Build history of the part. All positions in model axes, mm. Face numbers are marked on the shaded views. A direction names the side the tool comes from. Give positions to 0.01 mm unless a question says otherwise; leave off trailing zeros. Write each loop counter-clockwise with the first axis right and the second up, starting at its lowest first coordinate (ties: lowest second). Pieces come first, ordered by that corner, then holes. Notation, with made-up numbers: (-27, 1) -> (-11, 1) arc R36 ccw to (-11, 35) -> close; hole circle Ø7 at (34.25, -26.5). An arc over 180 degrees is marked (long way). Write item = value, one per line. Start each with the question number.
Q1. Saw through at A-A, the plane z = 0. List the corners of the cut face in (x, y).
Q2. Drop flat-ended pins along their axis: P1, Ø2, axis at x = 6.5, z = 0.5, coming from the -Y side; P2, Ø3, axis at x = 3, z = 0, coming from the +Y side; P3, Ø3, axis at y = 0, z = -1.5, coming from the +X side; P4, Ø2, axis at x = 6, y = 0, coming from the +Z side. Give the stop position or say it passes through.
Q3. Saw through at C-C, the plane x = 7. List the corners of the cut face in (y, z).
Q4. Mould opens along X. For the marked faces 1, 2, 3 and 4 say: pulls with the +X half, pulls with the -X half, needs draft (parallel to the pull), parting line crosses it, or undercut.
Q5. Saw through at B-B, the plane y = 0. List the corners of the cut face in (x, z), then the cut area to 3 significant figures.
Q6. Wall check: line 1 (X direction, y = 0.25, z = 1.05); line 2 (X direction, y = 0.05, z = 2.05); line 3 (Z direction, x = 3.25, y = 0.1). Give the ranges that are in metal, low to high.
Q7. Tool access for the marked faces 5 and 6: list every direction of +Z, -Z, +X, -X, +Y, -Y with a clear straight run to the whole face (end or side of a thin tool).
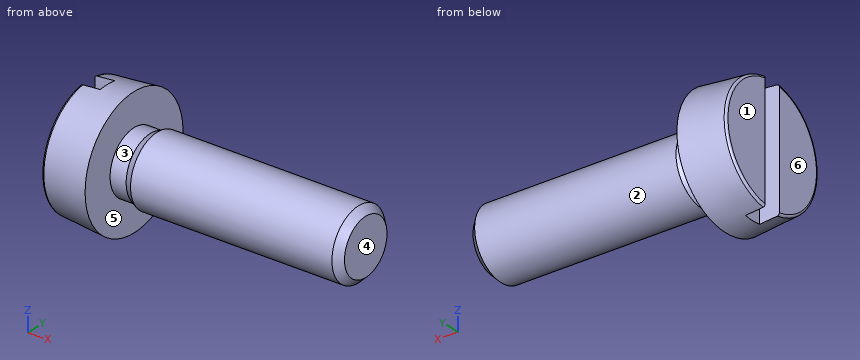
Autodesk Inventor part; units mm, degrees
ref_plane "Work Plane1" through (30.1625, 0, 0) normal (0, 0, -1) x (1, 0, 0)
ref_plane "YZ Plane" through (0, 0, 0) normal (1, 0, 0) x (0, 1, 0)
ref_plane "XZ Plane" through (0, 0, 0) normal (0, 1, 0) x (-1, 0, 0)
sketch "Szkic1" plane through (0, 0, 0) normal (0, 0, 1) x (1, 0, 0)
  line L0 (-2, 0) -> (10, 0)
  line L1 (10, 0) -> (10, 1.5)
  line L2 (10, 1.5) -> (1, 1.5)
  line L3 (1, 1.5) -> (0.6932, 1.3467)
  line L4 (0.6932, 1.3467) -> (0, 1.3467)
  line L5 (0, 1.3467) -> (0, 2.75)
  line L6 (-4.4, 0) -> (12.4, 0)
  line L7 (0, -0.55) -> (0, 3.3)
  line L8 (-2, 0) -> (-2, 2.575)
  line L9 (0, 2.75) -> (-2, 2.575)
  line L10 (1, 1.5) -> (0, 1.5) construction
  dimension "d0" = 10
  dimension "d1" = 9
  dimension "d2" = 0.3068
  dimension "d3" = 2
  dimension "d4" = 3
  dimension "d5" = 2.6935
  dimension "d9" = 5.5
  dimension "d10" = 5
revolve "Bryła" add sketch "Szkic1" angle 360 about axis through (-2, 0, 0) along (1, 0, 0)
sketch "Szkic2" plane through (-2, 0, 0) normal (-1, 0, 0) x (0, 0, 1)
  circle A0 centre (0, 0) radius 2.75
  line L0 (0, 0) -> (0, 2.575)
  line L1 (-2.75, 0.4) -> (2.75, 0.4)
  line L2 (2.75, 0.4) -> (2.75, -0.4)
  line L3 (2.75, -0.4) -> (-2.75, -0.4)
  line L4 (-2.75, -0.4) -> (-2.75, 0.4)
  line L5 (-2.75, 0) -> (2.75, 0) construction
  line L6 (0, 0.4) -> (0, -0.4) construction
  dimension "d11" = 0.8
  dimension "d12" = 5.5
fillet "Zaokrąglenie1" radius 0.1 1 edges at (-2, -2.575, 0)
extrude "Szczelina" cut sketch "Szkic2" against normal blind 0.85 contours A0 L3 L1 | L2 L3 A0 | A0 L1 L2 | A0 L4 L1 | L3 L4 A0
thread "Gwint"
chamfer "Faza1" distance 0.3067 distance2 0.3068 1 edges at (10, -1.5, 0) measured on face at (10, 0.417, 0.2189)
ref_plane "Work Plane1" through (30.1625, 0, 0) normal (0, 0, -1) x (1, 0, 0)
equation "\"d11\" = SBR"
equation "\"d12\" = KOD"
equation "\"d14\" = RR"
equation "\"d19\" = STI"
equation "\"d15\" = GEL"
equation "\"d17\" = -0.5 * SPD + 0.5 * GD"
equation "\"d0\" = NLG"
equation "\"d1\" = GEL"
equation "\"d3\" = KOH"
equation "\"d4\" = GD"
equation "\"d5\" = BDM"
equation "\"d9\" = KOD"
equation "\"d10\" = KEWI"
equation "\"GD\" = NND"
equation "\"NLG\" = 10"
equation "\"GEL\" = 9"
equation "\"KOD\" = 5.5"
equation "\"KOH\" = 2"
equation "\"GAL\" = 0.61345 * PTC"
equation "\"SPD\" = NND - 1.2269 * PTC"
equation "\"BDM\" = 2.6935"
equation "\"GUL\" = 0.61345 * PTC"
equation "\"RR\" = 0.1"
equation "\"SBR\" = 0.8"
equation "\"STI\" = 0.85"
equation "\"KEWI\" = 5deg"
equation "\"PTC\" = 0.5"
equation "\"THREADDIA\" = 3"
equation "\"TOA\" = 30deg"
equation "\"NND\" = 3"
equation "\"GD1\" = THREADDIA - 1.2269 * PTC"
properties part number "ISO 1207 - M3 x 10" material "Stal nierdzewna 440C"
Report:
q1.outline = (-2, -2.48) arc R0.1 ccw to (-1.91, -2.58) -> (0, -2.75) -> (0, -1.35) -> (0.69, -1.35) -> (1, -1.5) -> (9.69, -1.5) -> (10, -1.19) -> (10, 1.19) -> (9.69, 1.5) -> (1, 1.5) -> (0.69, 1.35) -> (0, 1.35) -> (0, 2.75) -> (-1.91, 2.58) arc R0.1 ccw to (-2, 2.48) -> (-2, 0.4) -> (-1.15, 0.4) -> (-1.15, -0.4) -> (-2, -0.4) -> close
q2.P1 = -1.5
q2.P2 = 1.5
q2.P3 = 10
q2.P4 = 1.5
q3.outline = circle Ø3 at (0, 0)
q4.face_1 = pulls with the -X half
q4.face_2 = needs draft
q4.face_3 = undercut
q4.face_4 = pulls with the +X half
q5.outline = (-1.15, -2.65) -> (0, -2.75) -> (0, -1.35) -> (0.69, -1.35) -> (1, -1.5) -> (9.69, -1.5) -> (10, -1.19) -> (10, 1.19) -> (9.69, 1.5) -> (1, 1.5) -> (0.69, 1.35) -> (0, 1.35) -> (0, 2.75) -> (-1.15, 2.65) -> close
q5.area = 35.9 mm2
q6.line_1 = -1.15 to 10
q6.line_2 = -1.15 to 0
q6.line_3 = -1.5 to 1.5
q7.face_5 = none
q7.face_6 = +Z, -Z, -X, +Y, -Y
